from build123d import *

# Parameters (mm, degrees)
F1_DEPTH       = 25
F5_D           = 5.5
F5_DEPTH       = 14.1
F5_TIP         = 1.6523667023
F5_ON_F3_D     = 5.5
F5_ON_F3_DEPTH = 14.1
F5_ON_F3_TIP   = 1.6523667023
F5_ON_F4_D     = 5.5
F5_ON_F4_DEPTH = 14.1
F5_ON_F4_TIP   = 1.6523667023
F6_W           = 1
F6_H           = 25
F7_DEPTH       = 30
F8_W           = 1
F8_H           = 25
F9_DEPTH       = 30


with BuildPart() as f1:
    # F0 (on Top) → F1 (new body)
    with BuildSketch(Plane.XY):
        with BuildLine():
            Line((-38.4127462552, -1.4693210872), (-63.4127462552, -1.4693210872))
            Line((-63.4127462552, -1.4693210872), (-63.4127462552, -11.4693210872))
            Line((-63.4127462552, -11.4693210872), (-43.749593064, -11.4693210872))
            ThreePointArc((-43.749593064, -11.4693210872), (-24.9127462552, -22.7959897839), (-6.0758994463, -11.4693210872))
            Line((-6.0758994463, -11.4693210872), (11.6210684322, -11.4693210872))
            ThreePointArc((11.6210684322, -11.4693210872), (30.0872537448, -22.4693210872), (48.5534390575, -11.4693210872))
            Line((48.5534390575, -11.4693210872), (66.0872537448, -11.4693210872))
            Line((66.0872537448, -11.4693210872), (66.0872537448, -1.4693210872))
            Line((66.0872537448, -1.4693210872), (41.0872537448, -1.4693210872))
            ThreePointArc((41.0872537448, -1.4693210872), (30.0872537448, -12.4693210872), (19.0872537448, -1.4693210872))
            Line((19.0872537448, -1.4693210872), (-11.4127462552, -1.4693210872))
            ThreePointArc((-11.4127462552, -1.4693210872), (-24.9127462552, -14.9693210872), (-38.4127462552, -1.4693210872))
        make_face()
    extrude(amount=F1_DEPTH)

    # F5
    with Locations(Plane.XZ.offset(11.4693210872)):
        with Locations((-53.5811696596, 12.5)):
            Hole(F5_D / 2, depth=F5_DEPTH)
            with Locations((0, 0, -(F5_DEPTH + F5_TIP / 2))):  # 118° drill point
                Cone(0, F5_D / 2, F5_TIP, mode=Mode.SUBTRACT)

    # F5 on F3
    with Locations(Plane.XZ.offset(11.4693210872)):
        with Locations((57.3203464011, 12.5)):
            Hole(F5_ON_F3_D / 2, depth=F5_ON_F3_DEPTH)
            with Locations((0, 0, -(F5_ON_F3_DEPTH + F5_ON_F3_TIP / 2))):  # 118° drill point
                Cone(0, F5_ON_F3_D / 2, F5_ON_F3_TIP, mode=Mode.SUBTRACT)

    # F5 on F4
    with Locations(Plane.XZ.offset(11.4693210872)):
        with Locations((2.772584493, 12.5)):
            Hole(F5_ON_F4_D / 2, depth=F5_ON_F4_DEPTH)
            with Locations((0, 0, -(F5_ON_F4_DEPTH + F5_ON_F4_TIP / 2))):  # 118° drill point
                Cone(0, F5_ON_F4_D / 2, F5_ON_F4_TIP, mode=Mode.SUBTRACT)

    # F6 (on face) → F7 (cut)
    with BuildSketch(Plane.YZ.offset(66.0872537448)):
        with Locations((-1.9693210872, 12.5)):
            Rectangle(F6_W, F6_H)
    extrude(amount=-F7_DEPTH, mode=Mode.SUBTRACT)

    # F8 (on face) → F9 (cut)
    with BuildSketch(Plane(origin=(-63.4127462552, 0, 0), x_dir=(0, -1, 0), z_dir=(-1, 0, 0))):
        with Locations((1.9693210872, 12.5)):
            Rectangle(F8_W, F8_H)
    extrude(amount=-F9_DEPTH, mode=Mode.SUBTRACT)


solid = f1.part
The listing builds one solid part. Answer for the finished solid, in the listing's coordinates (mm). A direction names the side the tool comes from. Round coordinates to 2 decimals unless told otherwise and drop trailing zeros. Order: outer loops, then holes, each group sorted by start corner. A loop starts at its lowest first (then second) coordinate and runs counter-clockwise, first axis right, second up. Notation, with made-up numbers: (42.5, 45) - (74.5, 45) arc R33 ccw to (74.5, 79) - close; hole circle Ø7 at (11.5, 45). An arc over 180 degrees is marked (long way). Write item = value, one per line. Start each with the question number.
1) Section C-C, the plane x = 4 is taken. Write down the section's boundary in (y, z), plus the area to 3 significant figures.
2) Straight lines are drawn through the part: L1, parallel to X at y = -5.75, z = 7; L2, parallel to X at y = -4.5, z = 18.5; L3, parallel to Y at x = -44, z = 5.5. For each, find the intervals that lie inside material, in ascending order.
3) For a pull along X with two mould halves and no side action, classify faces 4 (the flat face through (2.6, -11.469, 9.5)), 5 (the flat face through (-53.7, -11.469, 9.5)), 6 (the flat face through (-63.413, -7, 12)), 7 (the cylindrical face through (29.821, -12.466, 12.325)) as released by +X, released by -X, zero draft, split by the parting line, or undercut.
4) Section D-D, the plane y = -17.75 is taken. Write down the section's boundary in (x, z), plus the area to 3 significant figures.
5) Section A-A, the plane z = 12.5 is taken. Write down the section's boundary in (x, y).
6) For faces 1 (the flat face through (-48, -2.469, 12)), 2 (the flat face through (57.2, -11.469, 9.5)), 3 (the flat face through (54, -2.469, 12)), determine the directions among +Z, -Z, +X, -X, +Y, -Y from which every point of the face is accessible in a straight line to the end or side of a thin tool.
7) Given pin 1 (7 mm diameter, centred on x = 57.32, z = 12.5, fed in from +Y); pin 2 (5.5 mm diameter, centred on x = 60.5, z = 14.5, fed in from -Y); pin 3 (4 mm diameter, centred on y = -16, z = 18.5, fed in from +X), each flat-ended and moving along its own axis, determine where each tip first touches the part or whether it passes through.
8) Section B-B, the plane y = -8.75 is taken. Write down the section's boundary in (x, z), plus the area to 3 significant figures.
Results list:
q1.outline = (-11.47, 0) - (-1.47, 0) - (-1.47, 10.04) - (-11.47, 10.04) - close; (-11.47, 14.96) - (-1.47, 14.96) - (-1.47, 25) - (-11.47, 25) - close
q1.area = 201 mm^2
q2.L1 = -63.41 to -37.72, -12.11 to 19.95, 40.22 to 66.09
q2.L2 = -63.41 to -38.07, -11.76 to 19.51, 40.66 to 66.09
q2.L3 = -11.47 to -2.47
q3.face_4 = undercut
q3.face_5 = zero draft
q3.face_6 = released by -X
q3.face_7 = undercut
q4.outline = (-38.69, 0) - (-11.14, 0) - (-11.14, 25) - (-38.69, 25) - close; (16.82, 0) - (43.35, 0) - (43.35, 25) - (16.82, 25) - close
q4.area = 1,350 mm^2
q5.outline = (-63.41, -11.47) - (-56.33, -11.47) - (-56.33, -2.47) - (-63.41, -2.47) - close; (-50.83, -11.47) - (-43.75, -11.47) arc R21.33 ccw to (-6.08, -11.47) - (0.02, -11.47) - (0.02, -1.47) - (-11.41, -1.47) arc R13.5 cw to (-38.38, -2.47) - (-50.83, -2.47) - close; (5.52, -11.47) - (11.62, -11.47) arc R21 ccw to (48.55, -11.47) - (54.57, -11.47) - (54.57, -2.47) - (41.04, -2.47) arc R11 cw to (19.09, -1.47) - (5.52, -1.47) - close; (60.07, -11.47) - (66.09, -11.47) - (66.09, -2.47) - (60.07, -2.47) - close
q6.face_1 = +Z, -Z, -X, +Y
q6.face_2 = +Z, -Z, +X, -Y
q6.face_3 = +Z, -Z, +X, +Y
q7.pin_1 = -2.47
q7.pin_2 = -11.47
q7.pin_3 = 46.94
q8.outline = (-63.41, 0) - (-36.28, 0) - (-36.28, 25) - (-63.41, 25) - close; (-13.54, 0) - (21.84, 0) - (21.84, 25) - (-13.54, 25) - close; (38.33, 0) - (66.09, 0) - (66.09, 25) - (38.33, 25) - close; hole circle Ø5.5 at (-53.58, 12.5); hole circle Ø5.5 at (2.77, 12.5); hole circle Ø5.5 at (57.32, 12.5)
q8.area = 2,190 mm^2
